Geometry check sheet. Reference: the model listing, model coordinates, mm. A direction names the side the tool comes from. Round coordinates to 2 decimals unless told otherwise and drop trailing zeros. Order: outer loops, then holes, each group sorted by start corner. A loop starts at its lowest first (then second) coordinate and runs counter-clockwise, first axis right, second up. Notation, with made-up numbers: (-36.5, -27) - (11.5, -27) arc R18 cw to (11.5, -11) - close; hole circle Ø5 at (-6.5, -6.75). An arc over 180 degrees is marked (long way). Use a Markdown table: item, result. Add a question column.
(1) Thickness scan on line 1 along Z through (x, y) = (0, 14.3); line 2 along Y through (x, z) = (0.5, 106) (3 decimals); line 3 along Y through (x, z) = (-14.5, -114.3) (3 decimals). Record the ranges inside material, lowest first. Write a range as [from, to].
(2) Mould release check, pull along Z, two halves, no side actions. Record for faces 1 (the face through (0.54, 14.265, 100.677)), 2 (the face through (-0.628, -13.705, -32.155)), 3 (the face through (-14, 0, 127)), 4 (the face through (15.875, 0, -2)): released by +Z, released by -Z, zero draft, split by the parting line, or undercut.
(3) Section check B-B on z = 82.55. Record the boundary of the cut face in (x, y) (3 decimals).
(4) Section check A-A on z = -102.5. Record the boundary of the cut face in (x, y) (3 decimals).
(5) Gauge pin test, flat ends, axial feed: P1, Ø8, axis at y = 3.175, z = -40.132, coming from the +X side (3 decimals); P2, Ø1.5, axis at y = -7.5, z = 31, coming from the -X side; P3, Ø1.3, axis at x = 13.5, z = -16.5, coming from the +Y side (3 decimals); P4, Ø1.3, axis at x = -13.5, z = -18.5, coming from the -Y side (3 decimals). Record the tip position at first contact, or that the pin passes through.
(6) Access from +Z, -Z, +X, -X, +Y, -Y to the whole of each face (thin tool, end or side, straight path). Record for faces 5 (the face through (14.265, 3.284, 80.063)), 6 (the face through (-13.03, -0.07, 34.66)), 7 (the face through (-12.7, 0, -63)).
```python
from build123d import *

# Parameters (mm, degrees)
BOSS_EXTRUDE1_DEPTH           = 127
BOSS_EXTRUDE1_DEPTH_BACK      = 127
SKETCH3_W                     = 31.75
SKETCH3_H                     = 31.75
SKETCH3_W_2                   = 25.4
SKETCH3_H_2                   = 25.4
F_10_CLEARANCE_HOLE1_D        = 4.9784
SKETCH7_R                     = 14.2875
CUT_EXTRUDE1_DEPTH            = 7.62
CUT_EXTRUDE2_START            = -7.62
SKETCH8_R                     = 14.2875
CUT_EXTRUDE2_DEPTH            = 7.62
CUT_EXTRUDE3_DEPTH            = 132.867653824
F_10_CLEARANCE_HOLE2_D        = 4.9784
SKETCH13_R                    = 6.35
CUT_EXTRUDE4_DEPTH            = 132.867653824
TAP_DRILL_FOR_8_32_TAP1_D     = 3.4544
TAP_DRILL_FOR_8_32_TAP1_DEPTH = 5.08
TAP_DRILL_FOR_8_32_TAP1_TIP   = 1.037806461


with BuildPart() as part:
    # Sketch3 → Boss-Extrude1 (new, two sides: drawn at the far end of the back side and taken through both)
    with BuildSketch(Plane.XY.offset(-BOSS_EXTRUDE1_DEPTH_BACK)):
        Rectangle(SKETCH3_W, SKETCH3_H)
        Rectangle(SKETCH3_W_2, SKETCH3_H_2, mode=Mode.SUBTRACT)
    extrude(amount=BOSS_EXTRUDE1_DEPTH + BOSS_EXTRUDE1_DEPTH_BACK)

    # #10 Clearance Hole1 (through all)
    with Locations(Plane(origin=(0, 15.875, 0), x_dir=(1, 0, 0), z_dir=(0, 1, 0))):
        with Locations((-9.525, -117.475), (9.525, -117.475), (0, -98.247200001), (-7.111939052, -75.171256705)):
            Hole(F_10_CLEARANCE_HOLE1_D / 2)

    # Sketch7 → Cut-Extrude1 (cut)
    with BuildSketch(Plane(origin=(0, 15.875, 0), x_dir=(1, 0, 0), z_dir=(0, 1, 0))):
        with Locations(Location((0, 17.8816, 0), (0, 0, 270))):
            Circle(SKETCH7_R)
    extrude(amount=-CUT_EXTRUDE1_DEPTH, mode=Mode.SUBTRACT)

    # Sketch8 → Cut-Extrude2 (cut)
    with BuildSketch(Plane.XZ.offset(15.875).offset(CUT_EXTRUDE2_START)):
        with Locations(Location((0, -17.8816, 0), (0, 0, 90))):
            Circle(SKETCH8_R)
    extrude(amount=CUT_EXTRUDE2_DEPTH, mode=Mode.SUBTRACT)

    # Sketch9 → Cut-Extrude3 (cut, through all)
    with BuildSketch(Plane.XZ.offset(15.875)):
        with BuildLine():
            Line((-15.875, 34.663398263), (-15.875, 3.38353779))
            Line((-15.875, 3.38353779), (-12.7, 3.38353779))
            ThreePointArc((-12.7, 3.38353779), (-8.209871939, 5.243409729), (-6.35, 9.73353779))
            Line((-6.35, 9.73353779), (-6.883240315, 28.313398263))
            ThreePointArc((-6.883240315, 28.313398263), (-8.743112255, 32.803526323), (-13.233240315, 34.663398263))
            Line((-13.233240315, 34.663398263), (-15.875, 34.663398263))
        make_face()
    extrude(amount=-CUT_EXTRUDE3_DEPTH, mode=Mode.SUBTRACT)

    # #10 Clearance Hole2 (through all)
    with Locations(Plane(origin=(15.875, 0, 0), x_dir=(0, 0, -1), z_dir=(1, 0, 0))):
        with Locations((-82.55, 3.175), (114.3, 3.175), (40.132, 3.175)):
            Hole(F_10_CLEARANCE_HOLE2_D / 2)

    # Sketch13 → Cut-Extrude4 (cut, through all)
    with BuildSketch(Plane.XZ.offset(15.875)):
        with Locations((-20.955, 94.525686877)):
            Circle(SKETCH13_R)
    extrude(amount=-CUT_EXTRUDE4_DEPTH, mode=Mode.SUBTRACT)

    # Tap Drill for #8-32 Tap1
    with Locations(Plane(origin=(0, 15.875, 0), x_dir=(1, 0, 0), z_dir=(0, 1, 0))):
        with Locations((0, 35.9156), (0, -0.1524)):
            Hole(TAP_DRILL_FOR_8_32_TAP1_D / 2, depth=TAP_DRILL_FOR_8_32_TAP1_DEPTH)
            with Locations((0, 0, -(TAP_DRILL_FOR_8_32_TAP1_DEPTH + TAP_DRILL_FOR_8_32_TAP1_TIP / 2))):  # 118° drill point
                Cone(0, TAP_DRILL_FOR_8_32_TAP1_D / 2, TAP_DRILL_FOR_8_32_TAP1_TIP, mode=Mode.SUBTRACT)


solid = part.part
```
Check sheet entries:
| question | item | result |
|---|---|---|
| 1 | line 1 | z = [-127, -37.64], [-34.19, -32.17], [-3.59, -1.57], [1.88, 95.76], [100.74, 127] |
| 1 | line 2 | y = [-15.875, -12.7], [12.7, 15.875] |
| 1 | line 3 | y = [-15.875, 0.686], [5.664, 15.875] |
| 2 | face 1 | undercut |
| 2 | face 2 | undercut |
| 2 | face 3 | released by +Z |
| 2 | face 4 | zero draft |
| 3 | outline | (-15.875, -15.875) - (15.875, -15.875) - (15.875, 0.686) - (12.7, 0.686) - (12.7, -12.7) - (-12.7, -12.7) - (-12.7, 0.686) - (-15.875, 0.686) - close; (-15.875, 5.664) - (-12.7, 5.664) - (-12.7, 12.7) - (12.7, 12.7) - (12.7, 5.664) - (15.875, 5.664) - (15.875, 15.875) - (-15.875, 15.875) - close |
| 4 | outline | (-15.875, -15.875) - (15.875, -15.875) - (15.875, 15.875) - (-15.875, 15.875) - close; hole (-12.7, -12.7) - (12.7, -12.7) - (12.7, 12.7) - (-12.7, 12.7) - close |
| 5 | P1 | stops at x = 15.875 |
| 5 | P2 | stops at x = 12.7 |
| 5 | P3 | stops at y = 8.255 |
| 5 | P4 | stops at y = -8.255 |
| 6 | face 5 | +X, -X |
| 6 | face 6 | -X, +Y, -Y |
| 6 | face 7 | +Z, -Z |
